Verification items for the finished model (mm, model axes). Face numbers are marked on the shaded views. A direction names the side the tool comes from. Coordinates: 2 decimals unless noted, no trailing zeros. Loops run counter-clockwise (first coordinate to the right, second up) from the corner with the lowest first, then second, coordinate; pieces in that order, holes last. Notation, with made-up numbers: (80.25, 89) - (106.25, 89) arc R23 cw to (106.25, 104) - close; hole circle Ø11 at (85.25, 81). An arc over 180 degrees is marked (long way). Answer as CSV lines item,"result". Start each with the question number.
1. Set-up check for the marked faces 1, 2 and 3: record each of +Z, -Z, +X, -X, +Y, -Y from which the full face is reachable in a straight line by a thin tool's end or side.
2. Release check for a two-part mould opening along X. For the marked faces 4, 5 and 6 record: pulls with the +X half, pulls with the -X half, needs draft (parallel to the pull), parting line crosses it, or undercut.
3. Cross-section at B-B (x = -43). Enter the section's corners in (y, z).
4. Gauge pin test, flat ends, axial feed: P1, Ø1, axis at x = -62, y = -38, coming from the -Z side; P2, Ø2, axis at x = 30, z = 3, coming from the -Y side; P3, Ø1.5, axis at x = -61.5, z = 3.5, coming from the +Y side; P4, Ø1, axis at x = -59, z = 7, coming from the -Y side. Record the tip position at first contact, or that the pin passes through.
5. Cross-section at D-D (y = -43.5). Enter the section's corners in (x, z), plus the area to 3 significant figures.
6. Cross-section at C-C (y = -27). Enter the section's corners in (x, z).
7. Material ranges on line 1 (X direction, y = -33.5, z = 7.75); line 2 (Y direction, x = -59, z = 8.5); line 3 (Y direction, x = -62.5, z = 7.5), recorded low to high. Write a range as [from, to].
8. Cross-section at A-A (z = 3). Enter the section's corners in (x, y).
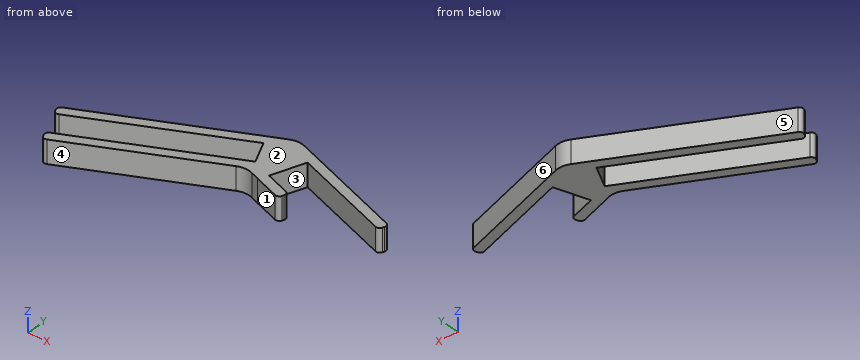
```python
from build123d import *

# Parameters (mm, degrees)
EXTRUDE_1_DEPTH = 12
FILLET_1_R      = 10
FILLET_2_R      = 10
FILLET_5_R      = 2
FILLET_6_R      = 2


with BuildPart() as part:
    # 草圖1 → 填料-伸長1 (new body)
    with BuildSketch(Plane.XY):
        Polygon((-89.273265788, -29.922645798), (0.928558352, 13.247145977), (66.944140174, -10.032522336), (65.138238425, -14.697469577), (13.313992743, 3.577780247), (7.327792319, -13.397655079), (21.473988424, -18.386155432), (19.835061436, -23.109984484), (4.845229239, -17.823985149), (-3.252616127, -14.806615195), (-79.583485532, -51.337891248), (-81.717667186, -46.81616648), (-3.242080184, -9.258447635), (-9.070002074, 2.918798623), (-87.320597555, -34.531241278), align=None)
    extrude(amount=EXTRUDE_1_DEPTH)

    # 圓角1
    fillet_1_edges = [part.edges().sort_by_distance(p)[0] for p in [
        (0.928558352, 13.247145977, 6),
    ]]
    fillet(fillet_1_edges, radius=FILLET_1_R)

    # 圓角2
    fillet_2_edges = [part.edges().sort_by_distance(p)[0] for p in [
        (-3.252616127, -14.806615195, 6),
    ]]
    fillet(fillet_2_edges, radius=FILLET_2_R)

    # 圓角5
    fillet_5_edges = [part.edges().sort_by_distance(p)[0] for p in [
        (65.138238425, -14.697469577, 6),
        (21.473988424, -18.386155432, 6),
        (19.835061436, -23.109984484, 6),
        (66.944140174, -10.032522336, 6),
    ]]
    fillet(fillet_5_edges, radius=FILLET_5_R)

    # 圓角6
    fillet_6_edges = [part.edges().sort_by_distance(p)[0] for p in [
        (-79.583485532, -51.337891248, 6),
        (-81.717667186, -46.81616648, 6),
        (-87.320597555, -34.531241278, 6),
        (-89.273265788, -29.922645798, 6),
    ]]
    fillet(fillet_6_edges, radius=FILLET_6_R)


solid = part.part
```
Values follow:
1,face 1,"+Z, -Z, -Y"
1,face 2,"+Z, +X, -X, +Y, -Y"
1,face 3,"+Z, -Z"
2,face 4,"undercut"
2,face 5,"pulls with the -X half"
2,face 6,"pulls with the +X half"
3,outline,"(-33.83, 0) - (-28.29, 0) - (-28.29, 12) - (-33.83, 12) - close; (-13.32, 0) - (-7.78, 0) - (-7.78, 12) - (-13.32, 12) - close"
4,P1,"stops at z = 0"
4,P2,"stops at y = -2.66"
4,P3,"stops at y = -16.27"
4,P4,"stops at y = -41.73"
5,outline,"(-74.79, 0) - (-63.21, 0) - (-63.21, 12) - (-74.79, 12) - close"
5,area,"139 mm²"
6,outline,"(-83.17, 0) - (-71.58, 0) - (-71.58, 12) - (-83.17, 12) - close; (-40.31, 0) - (-28.73, 0) - (-28.73, 12) - (-40.31, 12) - close"
7,line 1,"x = [-87.39, -85.17], [-53.89, -42.31]"
7,line 2,"y = [-41.49, -35.94], [-20.98, -15.43]"
7,line 3,"y = [-43.16, -37.62], [-22.65, -17.11]"
8,outline,"(-88.53, -31.68) - (-88.14, -32.6) arc R2 ccw to (-85.43, -33.63) - (-9.07, 2.92) - (-3.24, -9.26) - (-79.92, -45.96) arc R2 ccw to (-80.87, -48.62) - (-80.44, -49.52) arc R2 ccw to (-77.77, -50.47) - (-7.08, -16.64) arc R10 cw to (0.73, -16.29) - (4.85, -17.82) - (17.94, -22.44) arc R2 ccw to (20.49, -21.21) - (20.82, -20.27) arc R2 ccw to (19.6, -17.72) - (7.33, -13.4) - (13.31, 3.58) - (63.31, -14.05) arc R2 ccw to (65.84, -12.89) - (66.2, -11.96) arc R2 ccw to (65, -9.35) - (4.83, 11.87) arc R10 ccw to (-2.81, 11.46) - (-87.55, -29.1) arc R2 ccw to start"
